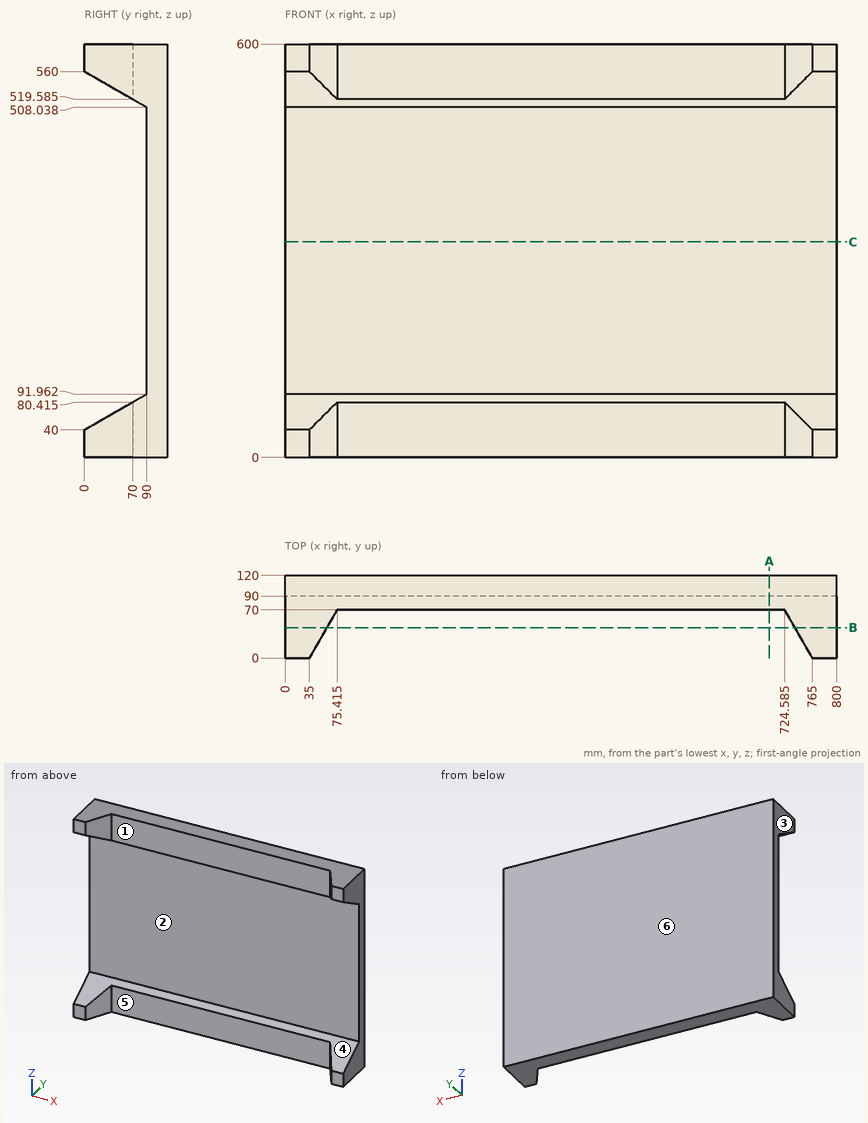
Can you work these out from the drawing? Everything is in mm from the part's minimum corner. A direction names the side the tool comes from. Give positions to 0.01 mm unless a question says otherwise; leave off trailing zeros. Order: outer loops, then holes, each group sorted by start corner. A loop starts at its lowest first (then second) coordinate and runs counter-clockwise, first axis right, second up. Notation, with made-up numbers: M 58,-8.5 L 113,-8.5 A13 cw 113,2.5 Z; hole C 58.25,-37.75 d4. An arc over 180 degrees is marked long. Use a Markdown table: item, result. Add a question column.
Item 1: Suppose I cut it at C-C (z = 313). List the corners of the cut face in (x, y) for me.
Item 2: Suppose I cut it at B-B (y = 44.5). List the corners of the cut face in (x, z) for me.
Item 3: Suppose I cut it at A-A (x = 702.5). List the corners of the cut face in (y, z) for me (1 decimal), then the cut area to 3 significant figures.
Item 4: If I drill on L1, parallel to Z at x = 726, y = 70 (1 decimal); L2, parallel to Y at x = 675.5, z = 155; L3, parallel to Z at x = 106.5, y = 84, over which ranges is the centre line in solid material (lowest first)? Write a range as [from, to].
Item 5: For the marked faces 4, 5 and 6, which set-ups out of +Z, -Z, +X, -X, +Y, -Y let a thin tool reach every point of the face, with its end or its side?
Item 6: Will these pins go through, and if not, where does the flat tip stop? pin 1 (12 mm diameter, centred on x = 603, z = 208.5, fed in from -Y); pin 2 (24 mm diameter, centred on x = 406, z = 47, fed in from -Y).
Item 7: We'd pull the mould along X, two halves only. Please class the marked faces 1, 2 and 3: +X half, -X half, draft (parallel to the pull), parting line (faces both ways), or undercut.
Answer sheet:
| question | item | result |
|---|---|---|
| 1 | outline | M 0,90 L 800,90 L 800,120 L 0,120 Z |
| 2 | outline | M 0,0 L 60.69,0 L 60.69,65.69 L 0,65.69 Z; M 0,534.31 L 60.69,534.31 L 60.69,600 L 0,600 Z; M 739.31,0 L 800,0 L 800,65.69 L 739.31,65.69 Z; M 739.31,534.31 L 800,534.31 L 800,600 L 739.31,600 Z |
| 3 | outline | M 70,0 L 120,0 L 120,600 L 70,600 L 70,519.6 L 90,508 L 90,92 L 70,80.4 Z |
| 3 | area | 21,400 mm² |
| 4 | L1 | z = [0, 80.4], [519.6, 600] |
| 4 | L2 | y = [90, 120] |
| 4 | L3 | z = [0, 88.5], [511.5, 600] |
| 5 | face 4 | +X, -X, -Y |
| 5 | face 5 | +Z, -Z, -Y |
| 5 | face 6 | +Z, -Z, +X, -X, +Y |
| 6 | pin 1 | stops at y = 90 |
| 6 | pin 2 | stops at y = 70 |
| 7 | face 1 | undercut |
| 7 | face 2 | draft |
| 7 | face 3 | -X half |
